Check sheet for the modelled part. Datum: model origin and axes. Units: mm. A direction names the side the tool comes from. Coordinates: 2 decimals unless noted, no trailing zeros. Use one line per item in the form item = value.
from build123d import *

# Parameters (mm, degrees)
SKETCH1_W           = 44.45
SKETCH1_H           = 19.05
BOSS_EXTRUDE1_DEPTH = 1.27
SKETCH2_R           = 7.9375
SKETCH2_R_2         = 6.35
BOSS_EXTRUDE2_DEPTH = 9.525
SKETCH4_W           = 9.525
SKETCH4_H           = 1.5875
BOSS_EXTRUDE3_DEPTH = 1.5875
SKETCH5_R           = 0.396875
BOSS_EXTRUDE4_DEPTH = 6.35
BOSS_EXTRUDE5_DEPTH = 3.175


with BuildPart() as part:
    # Sketch1 → Boss-Extrude1 (new body)
    with BuildSketch(Plane.XY):
        Rectangle(SKETCH1_W, SKETCH1_H)
    extrude(amount=BOSS_EXTRUDE1_DEPTH)

    # Sketch2 → Boss-Extrude2 (add)
    # profile 1 of 2: a face of its own
    with BuildSketch(Plane.XY.offset(1.27)):
        with Locations(Location((12.7, 0, 0), (0, 0, 180))):
            Circle(SKETCH2_R)
        with Locations(Location((12.7, 0, 0), (0, 0, 180))):
            Circle(SKETCH2_R_2, mode=Mode.SUBTRACT)
    # profile 2 of 2: a face of its own
    with BuildSketch(Plane.XY.offset(1.27)):
        with Locations(Location((-12.7, 0, 0), (0, 0, 180))):
            Circle(SKETCH2_R)
        with Locations(Location((-12.7, 0, 0), (0, 0, 180))):
            Circle(SKETCH2_R_2, mode=Mode.SUBTRACT)
    extrude(amount=BOSS_EXTRUDE2_DEPTH)

    # Sketch4 → Boss-Extrude3 (add)
    with BuildSketch(Plane(origin=(0, 0, 0), x_dir=(-1, 0, 0), z_dir=(0, 0, -1))):
        with Locations((-0.089489862, -8.73125)):
            Rectangle(SKETCH4_W, SKETCH4_H)
    extrude(amount=BOSS_EXTRUDE3_DEPTH)

    # Sketch5 → Boss-Extrude4 (add)
    with BuildSketch(Plane.XZ.offset(9.525)):
        with Locations(Location((-3.548073308, -0.79375, 0), (0, 0, 90))):
            Circle(SKETCH5_R)
        with Locations(Location((-1.008073308, -0.79375, 0), (0, 0, 90))):
            Circle(SKETCH5_R)
        with Locations(Location((1.531926692, -0.79375, 0), (0, 0, 90))):
            Circle(SKETCH5_R)
        with Locations(Location((4.071926692, -0.79375, 0), (0, 0, 90))):
            Circle(SKETCH5_R)
    extrude(amount=BOSS_EXTRUDE4_DEPTH)

    # Sketch6 → Boss-Extrude5 (add)
    with BuildSketch(Plane.XY.offset(1.27)):
        with BuildLine():
            Line((-3.175, 9.254970204), (3.175, 9.254970204))
            ThreePointArc((3.175, 9.254970204), (4.7625, 7.667470204), (3.175, 6.079970204))
            Line((3.175, 6.079970204), (-3.175, 6.079970204))
            ThreePointArc((-3.175, 6.079970204), (-4.7625, 7.667470204), (-3.175, 9.254970204))
        make_face()
    extrude(amount=BOSS_EXTRUDE5_DEPTH)


solid = part.part
(1) Mould release check, pull along X, two halves, no side actions. Record for faces 1 (the flat face through (0, 0, 1.27)), 2 (the flat face through (0, -7.937, -1)), 3 (the flat face through (-22.225, 0, 1)): +X half, -X half, draft (parallel to the pull), parting line (faces both ways), or undercut.
Established:
face_1 = undercut
face_2 = draft
face_3 = -X half
(2) Section check A-A, the plane z = 6.75. Give the number of separate pieces and of enclosed holes in the cut face, plus the area to 3 significant figures.
Established:
separate_pieces = 2
enclosed_holes = 2
area = 143 mm²
(3) Tool access check on faces 4 (the flat face through (0, 9.255, 3)), 5 (the flat face through (-4.673, -9, -1)), 6 (the flat face through (4.852, -9, -1)), 7 (the cylindrical face through (-20.271, -2.384, 5.966)), 8 (the flat face through (0, 8, 4.445)). Record the directions out of +Z, -Z, +X, -X, +Y, -Y that give a thin tool (end or side, any length) a straight path to the whole face; none if there is none.
Established:
face_4 = +Z, +X, -X, +Y
face_5 = -Z, -X, +Y, -Y
face_6 = -Z, +X, +Y, -Y
face_7 = +Z
face_8 = +Z, +Y, -Y
(4) Scan lines: line 1 along Y through (x, z) = (12.7, 4.5); line 2 along X through (y, z) = (1.5, 2.5); line 3 along Z through (x, y) = (12, -6.5) (3 decimals). Record each from-to range of solid material in increasing order.
Established:
line_1 = -7.94 to -6.35, 6.35 to 7.94
line_2 = -20.49 to -18.87, -6.53 to -4.91, 4.91 to 6.53, 18.87 to 20.49
line_3 = 0 to 10.795
(5) Go/stop test with flat-tipped pins: P1, Ø1, axis at x = 0, z = 3, coming from the +Y side (3 decimals); P2, Ø1, axis at x = 2.5, z = 1, coming from the -Y side (3 decimals); P3, Ø1, axis at y = 3, z = 8.5, coming from the +X side. Record where each tip stops, or that it passes through.
Established:
P1 = 9.255
P2 = -9.525
P3 = 20.23
